from build123d import *

# Parameters (mm, degrees)
SKETCH1_R               = 28.575
BOSS_EXTRUDE1_DEPTH     = 25
BOSS_EXTRUDE1_DRAFT     = -45
SKETCH3_R               = 53.575
BOSS_EXTRUDE2_DEPTH     = 60
CUT_EXTRUDE1_DEPTH      = 114.866418447
CUT_EXTRUDE1_DEPTH_BACK = 114.866418447
SKETCH4_R               = 19.05


with BuildPart() as part:
    # Sketch1 → Boss-Extrude1 (with draft: the straight prism first)
    with BuildSketch(Plane.XY):
        Circle(SKETCH1_R)
    extrude(amount=BOSS_EXTRUDE1_DEPTH)
    # Boss-Extrude1: the draft: its side faces are tilted about the plane it starts from
    boss_extrude1_sides = [part.faces().sort_by_distance(p)[0] for p in [
        (-28.575, 0, 12.5),
    ]]
    draft(boss_extrude1_sides, Plane.XY, BOSS_EXTRUDE1_DRAFT)

    # Sketch3 → Boss-Extrude2 (add)
    with BuildSketch(Plane.XY.offset(25)):
        Circle(SKETCH3_R)
    extrude(amount=BOSS_EXTRUDE2_DEPTH)

    # Sketch4 → Cut-Extrude1 (cut, two sides: drawn at the far end of the back side and taken through both)
    with BuildSketch(Plane(origin=(0, 0, 0), x_dir=(0, 0, -1), z_dir=(1, 0, 0)).offset(-CUT_EXTRUDE1_DEPTH_BACK)):
        with Locations((-55, 0)):
            Circle(SKETCH4_R)
    extrude(amount=CUT_EXTRUDE1_DEPTH + CUT_EXTRUDE1_DEPTH_BACK, mode=Mode.SUBTRACT)


solid = part.part
Work out the finished part from the listing and answer in its coordinate system (mm). Round coordinates to 2 decimals unless told otherwise and drop trailing zeros. Write each loop counter-clockwise with the first axis right and the second up, starting at its lowest first coordinate (ties: lowest second). Pieces come first, ordered by that corner, then holes. Notation, with made-up numbers: (39, 33) -> (98, 33) arc R12 ccw to (98, 55) -> close; hole circle Ø8 at (85.5, 68.5). An arc over 180 degrees is marked (long way). Answer as CSV lines item,"result". Start each with the question number.
(1) The part is cut by section B-B, the plane y = 0. Give the vertices of the cut face in (x, z) (3 decimals), then the cut area to 3 significant figures.
(2) Each of these flat-tipped pins is pushed along its axis until it touches: pin 1 (10 mm diameter, centred on x = -13, z = 14, fed in from +Y); pin 2 (3 mm diameter, centred on x = 2, z = 18.5, fed in from -Y); pin 3 (8 mm diameter, centred on y = 28.5, z = 31.5, fed in from +X). Where does it stop, or does it pass through?
(3) The part is cut by section C-C, the plane z = 55. Give the vertices of the cut face in (x, y) (3 decimals), then the cut area to 3 significant figures.
(4) The mould has two halves that part along Y. Classify faces 1 (the flat face through (-1, 1, 85)), 2 (the cylindrical face through (-0.75, -18.597, 59.13)), 3 (the cylindrical face through (49.49, -20.52, 54.58)): +Y half, -Y half, draft (parallel to the pull), parting line (faces both ways), or undercut.
(5) The part is cut by section D-D, the plane z = 76. Give the vertices of the cut face in (x, y) (3 decimals).
(6) Find the intervals of material crossed by probe 1 along Z at (x, y) = (6, 0); probe 2 along Y at (x, z) = (-0.5, 54); probe 3 along Z at (x, y) = (-40, 0) (3 decimals), in increasing order.
(7) The part is cut by section A-A, the plane x = 0. Give the vertices of the cut face in (y, z) (3 decimals), then the cut area to 3 significant figures.
Output values:
1,outline,"(-53.575, 25) -> (-28.575, 0) -> (28.575, 0) -> (53.575, 25) -> (53.575, 35.95) -> (-53.575, 35.95) -> close; (-53.575, 74.05) -> (53.575, 74.05) -> (53.575, 85) -> (-53.575, 85) -> close"
1,area,"4,400 mm²"
2,pin 1,"stops at y = 45.94"
2,pin 2,"stops at y = -48.54"
2,pin 3,"stops at x = 47.64"
3,outline,"(-50.074, -19.05) arc R53.575 ccw to (50.074, -19.05) -> close; (-50.074, 19.05) -> (50.074, 19.05) arc R53.575 ccw to start"
3,area,"5,020 mm²"
4,face 1,"draft"
4,face 2,"undercut"
4,face 3,"parting line"
5,outline,"circle Ø107.15 at (0, 0)"
6,probe 1,"z = 0 to 35.95, 74.05 to 85"
6,probe 2,"y = -53.57 to -19.02, 19.02 to 53.57"
6,probe 3,"z = 11.425 to 35.95, 74.05 to 85"
7,outline,"(-53.575, 25) -> (-28.575, 0) -> (28.575, 0) -> (53.575, 25) -> (53.575, 85) -> (-53.575, 85) -> close; hole circle Ø38.1 at (0, 55)"
7,area,"7,340 mm²"
